Geometry: final body of the model. Coordinates: model frame, mm. A direction names the side the tool comes from. Round coordinates to 2 decimals unless told otherwise and drop trailing zeros. Loops run counter-clockwise (first coordinate to the right, second up) from the corner with the lowest first, then second, coordinate; pieces in that order, holes last. Notation, with made-up numbers: (1.25, 26) - (28.25, 26) arc R30 ccw to (28.25, 51) - close; hole circle Ø6 at (-15, 3). An arc over 180 degrees is marked (long way). Answer as CSV lines item,"result".
from build123d import *

# Parameters (mm, degrees)
F1_DEPTH       = 6
F3_D           = 3
F3_CSINK_D     = 4
F3_CSINK_ANGLE = 90


# Not quite as in the source:
# - a feature names something its author has since deleted; it is built from what else it names


with BuildPart() as f1:
    # F0 (on Front) → F1 (new body)
    with BuildSketch(Plane.XZ):
        with BuildLine():
            Line((12.5, -2.1), (12.5, 0))
            ThreePointArc((12.5, 0), (11.2405591591, 3.0405591591), (8.2, 4.3))
            Line((8.2, 4.3), (0, 4.3))
            Line((0, 4.3), (0, -2.1))
            Line((0, -2.1), (6.3, -2.1))
            Line((6.3, -2.1), (6.3, 0))
            ThreePointArc((6.3, 0), (8.2, 1.9), (10.1, 0))
            Line((10.1, 0), (10.1, -2.1))
            Line((10.1, -2.1), (12.5, -2.1))
        make_face()
    extrude(amount=F1_DEPTH)

    # F3 (through all)
    with Locations(Plane.XY.offset(4.3)):
        with Locations((3.15, -3)):
            CounterSinkHole(F3_D / 2, F3_CSINK_D / 2, counter_sink_angle=F3_CSINK_ANGLE)


solid = f1.part
(1) Pin query (flat end, axial travel): P1, Ø2.5, axis at x = 3.15, y = -3, coming from the +Z side. Return the tip coordinate at first contact, or that it passes through.
Findings below:
P1,"through"
(2) Section D-D (y = -5.4). Output: boundary loops of the cut face in (x, z), and give its area (3 significant figures).
Findings below:
outline,"(0, -2.1) - (6.3, -2.1) - (6.3, 0) arc R1.9 cw to (10.1, 0) - (10.1, -2.1) - (12.5, -2.1) - (12.5, 0) arc R4.3 ccw to (8.2, 4.3) - (0, 4.3) - close"
area,"62.4 mm2"
(3) Draft query along Y for faces 3 (the face through (11.27, -2.96, 3.01)), 4 (the face through (1.72, -2.55, 0.81)), 5 (the face through (6, -6, 1)), 6 (the face through (6, 0, 1)). Return one class per face: pulls with the +Y half, pulls with the -Y half, needs draft (parallel to the pull), parting line crosses it, or undercut.
Findings below:
face 3,"needs draft"
face 4,"undercut"
face 5,"pulls with the -Y half"
face 6,"pulls with the +Y half"
(4) Material intervals for line 1 along X through (y, z) = (-3, -0.25); line 2 along Y through (x, z) = (3.15, -0.6); line 3 along X through (y, z) = (-1.75, 2.25), sorted ascending.
Findings below:
line 1,"0 to 1.65, 4.65 to 6.3, 10.1 to 12.5"
line 2,"-6 to -4.5, -1.5 to 0"
line 3,"0 to 2.32, 3.98 to 11.86"
(5) Access query for faces 1 (the face through (12.5, -3, -1)), 2 (the face through (6.3, -3, -1)). Directions: +Z, -Z, +X, -X, +Y, -Y. A direction counts if a zero-diameter tool reaches every point of the face in a straight line with its end or side. Return the directions, or none.
Findings below:
face 1,"+Z, -Z, +X, +Y, -Y"
face 2,"-Z, +Y, -Y"
(6) Section B-B (y = -3). Output: boundary loops of the cut face in (x, z), and give its area (3 significant figures).
Findings below:
outline,"(0, -2.1) - (1.65, -2.1) - (1.65, 3.8) - (1.15, 4.3) - (0, 4.3) - close; (4.65, -2.1) - (6.3, -2.1) - (6.3, 0) arc R1.9 cw to (10.1, 0) - (10.1, -2.1) - (12.5, -2.1) - (12.5, 0) arc R4.3 ccw to (8.2, 4.3) - (5.15, 4.3) - (4.65, 3.8) - close"
area,"42.9 mm2"
(7) Section A-A (z = -1). Output: boundary loops of the cut face in (x, y), and give its area (3 significant figures).
Findings below:
outline,"(0, -6) - (6.3, -6) - (6.3, 0) - (0, 0) - close; (10.1, -6) - (12.5, -6) - (12.5, 0) - (10.1, 0) - close; hole circle Ø3 at (3.15, -3)"
area,"45.1 mm2"
(8) Section C-C (x = 3.15). Output: boundary loops of the cut face in (y, z).
Findings below:
outline,"(-6, -2.1) - (-4.5, -2.1) - (-4.5, 3.8) - (-5, 4.3) - (-6, 4.3) - close; (-1.5, -2.1) - (0, -2.1) - (0, 4.3) - (-1, 4.3) - (-1.5, 3.8) - close"
